Can you work these out from the drawing? Everything is in mm from the part's minimum corner. A direction names the side the tool comes from. Coordinates: 2 decimals unless noted, no trailing zeros. Order: outer loops, then holes, each group sorted by start corner. A loop starts at its lowest first (then second) coordinate and runs counter-clockwise, first axis right, second up. Notation, with made-up numbers: (30.5, 62) - (87.5, 62) arc R24 cw to (87.5, 79) - close; hole circle Ø9 at (-19.5, -23). An arc over 180 degrees is marked (long way). Use a Markdown table: item, result. Add a question column.
(1) If I drill on L1, parallel to Z at x = 3.9, y = 9.5 (1 decimal); L2, parallel to Z at x = 2.6, y = 6.5; L3, parallel to Y at x = 5.75, z = 2.15 (1 decimal), over which ranges is the centre line in solid material (lowest first)? Write a range as [from, to].
(2) I want a section at A-A (y = 6.75). List the corners of the cut face in (x, z) for me.
(3) On a 3-axis mill with a long thin cutter (end or side, diameter ignored), from which of +Z, -Z, +X, -X, +Y, -Y can I reach the whole of each face in a straight line? I mean the marked faces 1 and 2. Say none if no direction works.
(4) For pin 1 Ø2 at (x, y) = (4, 6.5) entering from -Z; pin 2 Ø2 at (x, y) = (1.5, 7.5) entering from -Z, each with a flat end and sliding along its axis, tell me the tip position at first contact or that it passes through.
(5) We'd pull the mould along X, two halves only. Please class the marked faces 3, 4, 5 and 6: pulls with the +X half, pulls with the -X half, needs draft (parallel to the pull), parting line crosses it, or undercut.
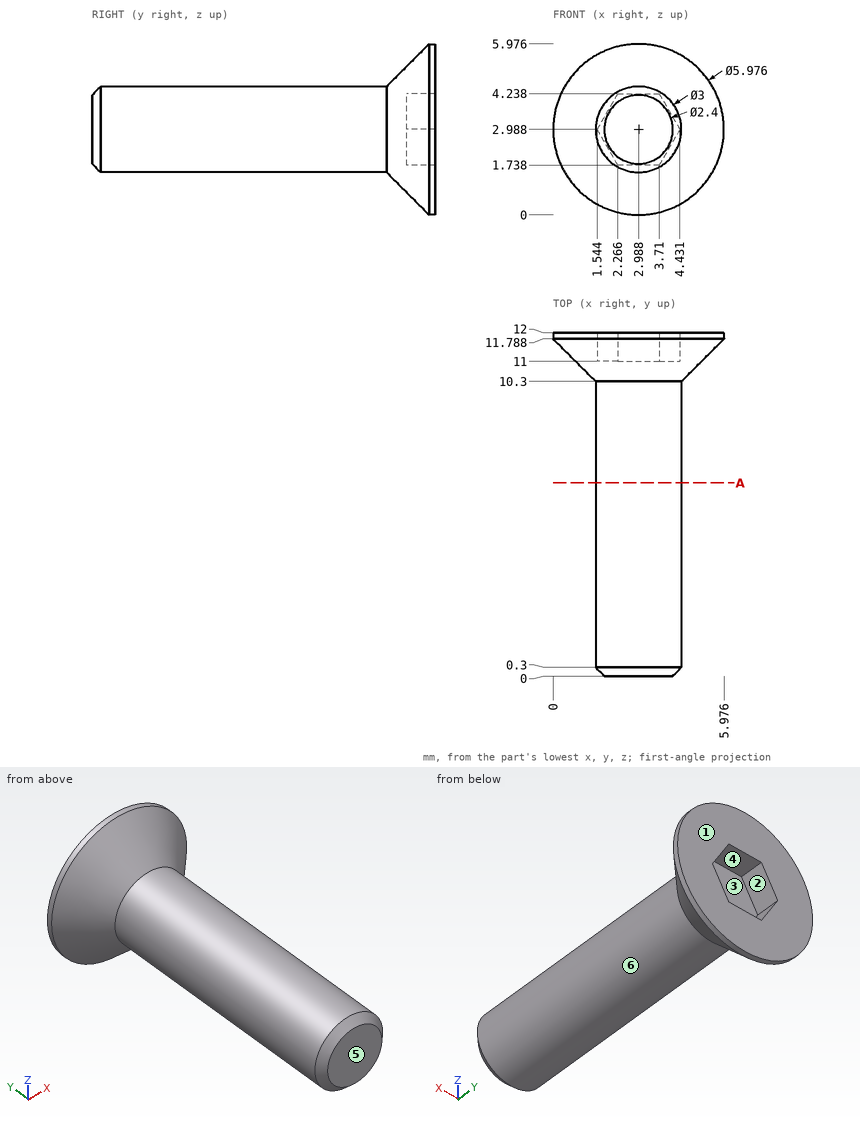
Answers follow:
| question | item | result |
|---|---|---|
| 1 | L1 | z = [1.8, 4.2] |
| 1 | L2 | z = [1.54, 4.44] |
| 1 | L3 | y = [11.7, 12] |
| 2 | outline | circle Ø3 at (2.99, 2.99) |
| 3 | face 1 | +Z, -Z, +X, -X, +Y |
| 3 | face 2 | +Y |
| 4 | pin 1 | stops at z = 1.49 |
| 4 | pin 2 | stops at z = 1.57 |
| 5 | face 3 | undercut |
| 5 | face 4 | undercut |
| 5 | face 5 | needs draft |
| 5 | face 6 | parting line crosses it |
